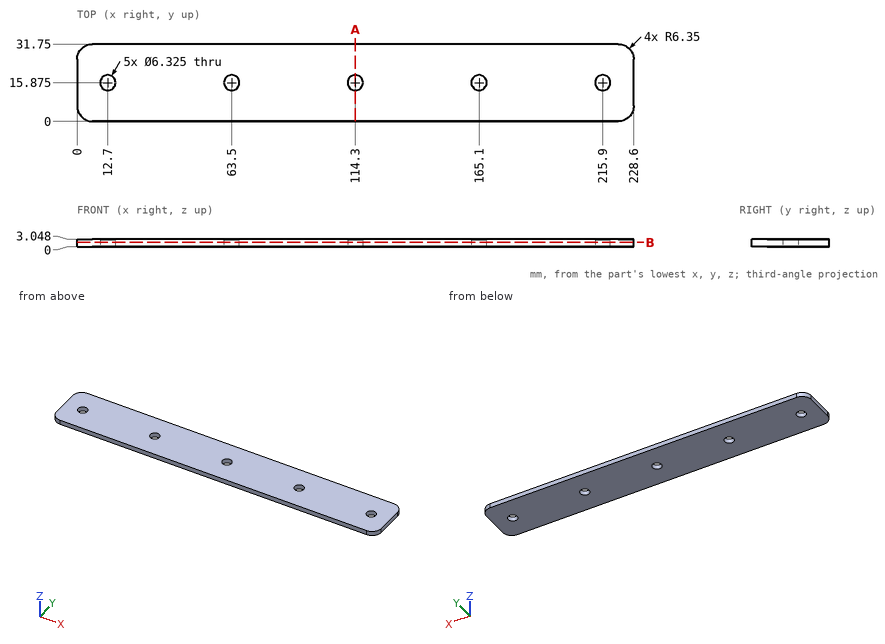
Geometry: see drawing. Coordinates: mm, zero at the bounding-box minimum. Round coordinates to 2 decimals unless told otherwise and drop trailing zeros. Loops run counter-clockwise (first coordinate to the right, second up) from the corner with the lowest first, then second, coordinate; pieces in that order, holes last. Notation, with made-up numbers: (56, 70.25) - (76, 70.25) arc R23 cw to (76, 109.25) - close; hole circle Ø9 at (-30.5, 8.5). An arc over 180 degrees is marked (long way). Use CSV: the item, a comma, the result in double quotes.
Q1. Pin query (flat end, axial travel): pin 1 Ø5.5 at (x, y) = (114.3, 15.875) entering from +Z. Return the tip coordinate at first contact, or that it passes through.
Reported:
pin 1,"through"
Q2. Section query A-A, the plane x = 114.3. Output: boundary loops of the cut face in (y, z).
Reported:
outline,"(0, 0) - (12.71, 0) - (12.71, 3.05) - (0, 3.05) - close; (19.04, 0) - (31.75, 0) - (31.75, 3.05) - (19.04, 3.05) - close"
Q3. Section query B-B, the plane z = 1.75. Give the number of separate pieces and of enclosed holes in the cut face, then the cut area to 3 significant figures.
Reported:
separate pieces,"1"
enclosed holes,"5"
area,"7,070 mm^2"
Q4. Ray query, line 1 along X through (y, z) = (16, 1.6); line 2 along X through (y, z) = (13, 2.7) (1 decimal); line 3 along Y through (x, z) = (165.1, 1.2). Return the intervals inside material, ascending.
Reported:
line 1,"0 to 9.54, 15.86 to 60.34, 66.66 to 111.14, 117.46 to 161.94, 168.26 to 212.74, 219.06 to 228.6"
line 2,"0 to 11.4, 14 to 62.2, 64.8 to 113, 115.6 to 163.8, 166.4 to 214.6, 217.2 to 228.6"
line 3,"0 to 12.71, 19.04 to 31.75"
